Verification items for the finished model (mm, model axes). A direction names the side the tool comes from. Coordinates: 2 decimals unless noted, no trailing zeros. Order: outer loops, then holes, each group sorted by start corner. A loop starts at its lowest first (then second) coordinate and runs counter-clockwise, first axis right, second up. Notation, with made-up numbers: M 6.5,-8 L 52.5,-8 A15 ccw 52.5,19 Z; hole C 15,74 d7. An arc over 180 degrees is marked long. Answer as a JSON object with one key per item and string values. Group by question number.
(1) Cross-section at B-B (y = -18.5). Enter the section's corners in (x, z).
(2) Access from +Z, -Z, +X, -X, +Y, -Y to the whole of each face (thin tool, end or side, straight path). Record for faces 4 (the face through (7.165, 10.626, -13.858)), 5 (the face through (1.693, -1.434, -22.435)).
(3) Cross-section at A-A (z = 0). Enter the section's corners in (x, y) (1 decimal).
(4) Material ranges on line 1 (Z direction, x = 1.75, y = -1); line 2 (Z direction, x = -4.25, y = 0); line 3 (X direction, y = 17, z = 10), recorded low to high.
(5) Gauge pin test, flat ends, axial feed: pin 1 Ø12.5 at (y, z) = (-19.08, -19.08) entering from -X; pin 2 Ø15.5 at (y, z) = (19.08, 19.08) entering from +X; pin 3 Ø6 at (x, y) = (-5.5, 21) entering from +Z. Record the tip position at first contact, or that the pin passes through.
(6) Cross-section at C-C (z = -30). Enter the section's corners in (x, y), plus the area to 3 significant figures.
(7) Mould release check, pull along Z, two halves, no side actions. Record for faces 1 (the face through (-3.162, 9, -10)), 2 (the face through (1.69, -14.85, 16.88)), 3 (the face through (-5.58, 12.4, -2.75)): released by +Z, released by -Z, zero draft, split by the parting line, or undercut.
from build123d import *

# Parameters (mm, degrees)
F2_R     = 4.77266
F3_DEPTH = 12.7
F4_COUNT = 8


with BuildPart() as f1:
    # F0 (on Front) → F1 (revolve)
    with BuildSketch(Plane.XZ):
        Polygon((-7.9375, 12.7), (-7.9375, 11.176), (7.9375, 11.176), (7.9375, 17.4625), (6.4135, 17.4625), (6.4135, 41.275), (-3.1623, 41.275), (-3.1623, 12.7), align=None)
    revolve(axis=Axis((0, 0, 0), (1, 0, 0)))

    # F2 (on Right) → F3 (cut, symmetric)
    with BuildSketch(Plane.YZ):
        with Locations((-26.9875, 0)):
            Circle(F2_R)
    f3 = extrude(amount=F3_DEPTH, both=True, mode=Mode.SUBTRACT)

    # F4: F3 ×8 about axis
    f4_axis = Axis((0, 0, 0), (1, 0, 0))
    for i in range(1, F4_COUNT):
        add(f3.rotate(f4_axis, i * 360 / F4_COUNT), mode=Mode.SUBTRACT)


solid = f1.part
Taken from the geometry:
{
 "1": {"outline": "M -3.16,-36.9 L 6.41,-36.9 L 6.41,-23.82 L -3.16,-23.82 Z; M -3.16,-14.35 L 6.41,-14.35 L 6.41,14.35 L -3.16,14.35 Z; M -3.16,23.82 L 6.41,23.82 L 6.41,36.9 L -3.16,36.9 Z"},
 "2": {"face 4": "+X", "face 5": "+X, -X"},
 "3": {"outline": "M -7.9,-12.7 L -3.2,-12.7 L -3.2,-22.2 L 6.4,-22.2 L 6.4,-17.5 L 7.9,-17.5 L 7.9,-11.2 L -7.9,-11.2 Z; M -7.9,11.2 L 7.9,11.2 L 7.9,17.5 L 6.4,17.5 L 6.4,22.2 L -3.2,22.2 L -3.2,12.7 L -7.9,12.7 Z; M -3.2,-41.3 L 6.4,-41.3 L 6.4,-31.8 L -3.2,-31.8 Z; M -3.2,31.8 L 6.4,31.8 L 6.4,41.3 L -3.2,41.3 Z"},
 "4": {"line 1": "z = -41.26 to -31.65, -22.32 to -11.13, 11.13 to 22.32, 31.65 to 41.26", "line 2": "z = -12.7 to -11.18, 11.18 to 12.7", "line 3": "x = -3.16 to 6.41"},
 "5": {"pin 1": "stops at x = -3.16", "pin 2": "stops at x = 6.41", "pin 3": "stops at z = 36.58"},
 "6": {"outline": "M -3.16,-28.35 L 6.41,-28.35 L 6.41,-3.7 L -3.16,-3.7 Z; M -3.16,3.7 L 6.41,3.7 L 6.41,28.35 L -3.16,28.35 Z", "area": "472 mm²"},
 "7": {"face 1": "zero draft", "face 2": "undercut", "face 3": "split by the parting line"}
}
